```python
from build123d import *

# Parameters (mm, degrees)
BOSS_EXTRUDE1_DEPTH = 6.35
FILLET1_R           = 3.175


with BuildPart() as part:
    # Sketch1 → Boss-Extrude1 (new body)
    with BuildSketch(Plane.XY):
        Polygon((0, 0), (-355.6, 0), (-304.8, 95.25), (-254, 95.25), align=None)
    extrude(amount=BOSS_EXTRUDE1_DEPTH)

    # Fillet1
    fillet1_edges = [part.edges().sort_by_distance(p)[0] for p in [
        (-330.2, 47.625, 6.35),
        (-330.2, 47.625, 0),
        (-127, 47.625, 6.35),
        (-127, 47.625, 0),
    ]]
    fillet(fillet1_edges, radius=FILLET1_R - 0.0001)  # a hair under: the kernel refuses the full size


solid = part.part
```
Could you check a few things on this model? Use its own coordinates, in mm. Round coordinates to 2 decimals unless told otherwise and drop trailing zeros. Write each loop counter-clockwise with the first axis right and the second up, starting at its lowest first coordinate (ties: lowest second). Pieces come first, ordered by that corner, then holes.
(1) Suppose I cut it at A-A on z = 5. Write out the boundary of the cut face in (x, y), and give its area (3 significant figures).
Findings below:
outline: (-354.95, 0) - (-1.64, 0) - (-255.64, 95.25) - (-304.15, 95.25) - close
area: 19,100 mm2
(2) If I drill on probe 1 along Z at (x, y) = (-245, 91.5); probe 2 along Z at (x, y) = (-333, 37.5); probe 3 along Y at (x, z) = (-55, 0.5), over which ranges is the centre line in solid material (lowest first)?
Findings below:
probe 1: z = 1.72 to 4.63
probe 2: z = 0.12 to 6.23
probe 3: y = 0 to 19.06
(3) For pin 1 (2 mm diameter, centred on x = -223.5, z = 3.5, fed in from +Y); pin 2 (1.5 mm diameter, centred on y = 73.5, z = 4, fed in from -X), each with a flat end and sliding along its axis, tell me the tip position at first contact or that it passes through.
Findings below:
pin 1: stops at y = 84.18
pin 2: stops at x = -316.72
